Geometry: final body of the model. Coordinates: model frame, mm. Face numbers are marked on the shaded views. Give positions to 0.01 mm unless a question says otherwise; leave off trailing zeros. Write each loop counter-clockwise with the first axis right and the second up, starting at its lowest first coordinate (ties: lowest second). Pieces come first, ordered by that corner, then holes. Notation, with made-up numbers: M -8.75,77.5 L 49.25,77.5 A3 cw 49.25,81.5 Z; hole C 75,-3 d11. An arc over 180 degrees is marked long. Use a Markdown table: item, result. Add a question column.
(1) Pin query (flat end, axial travel): pin 1 Ø6 at (x, y) = (1506.11, -138.7) entering from +Z (3 decimals); pin 2 Ø1 at (x, z) = (1473, 2) entering from +Y; pin 3 Ø1 at (x, z) = (1458.5, 8) entering from +Y; pin 4 Ø3 at (x, y) = (1506.11, -23.75) entering from +Z. Return the tip coordinate at first contact, or that it passes through.
(2) Cut plane B-B (y = -94.5). Output: boundary loops of the cut face in (x, z) (3 decimals), plus the area to 3 significant figures.
(3) Cut plane D-D (y = -14). Output: boundary loops of the cut face in (x, z) (3 decimals), plus the area to 3 significant figures.
(4) Cut plane A-A (z = 5.5). Output: boundary loops of the cut face in (x, y), plus the area to 3 significant figures.
(5) Draft query along Y for the marked faces 1 and 2. Return one class per face: released by +Y, released by -Y, zero draft, split by the parting line, or undercut.
(6) Material intervals for L1, parallel to Y at x = 1467.5, z = 2.25; L2, parallel to X at y = -38, z = 3; L3, parallel to Z at x = 1558, y = -60 (3 decimals), sorted ascending.
(7) Cut plane C-C (x = 1491.5). Output: boundary loops of the cut face in (y, z) (3 decimals).
```python
from build123d import *

# Parameters (mm, degrees)
SKETCH1_W           = 108.712
SKETCH1_H           = 108.712
SKETCH1_R           = 2.54
SKETCH1_R_2         = 3.175
SKETCH1_W_2         = 83.312
SKETCH1_H_2         = 83.312
SKETCH1_R_3         = 0.94996
SKETCH1_R_4         = 0.95
BOSS_EXTRUDE1_DEPTH = 3.175
SKETCH2_R           = 2.54
SKETCH2_R_2         = 0.95
BOSS_EXTRUDE2_DEPTH = 6.35
SKETCH3_R           = 2.54
BOSS_EXTRUDE3_DEPTH = 3.175


with BuildPart() as part:
    # Sketch1 → Boss-Extrude1 (new body)
    # profile 1 of 9: a face of its own
    with BuildSketch(Plane.XY):
        with Locations((1506.110862596, -71.75697427)):
            Rectangle(SKETCH1_W, SKETCH1_H)
        with Locations((1506.110862596, -23.75097427)):
            Circle(SKETCH1_R, mode=Mode.SUBTRACT)
        with Locations((1458.104862596, -23.75097427)):
            Circle(SKETCH1_R_2, mode=Mode.SUBTRACT)
        with Locations((1506.110862596, -119.76297427)):
            Circle(SKETCH1_R, mode=Mode.SUBTRACT)
        with Locations((1554.116862596, -71.75697427)):
            Circle(SKETCH1_R, mode=Mode.SUBTRACT)
        with Locations((1458.104862596, -71.75697427)):
            Circle(SKETCH1_R, mode=Mode.SUBTRACT)
        with Locations((1458.104862596, -119.76297427)):
            Circle(SKETCH1_R, mode=Mode.SUBTRACT)
        with Locations((1554.116862596, -119.76297427)):
            Circle(SKETCH1_R, mode=Mode.SUBTRACT)
        with Locations((1554.116862596, -23.75097427)):
            Circle(SKETCH1_R, mode=Mode.SUBTRACT)
        with Locations((1506.110862596, -71.75697427)):
            Rectangle(SKETCH1_W_2, SKETCH1_H_2, mode=Mode.SUBTRACT)
    # profile 2 of 9: a face of its own
    with BuildSketch(Plane.XY):
        with Locations((1554.116862596, -119.76297427)):
            Circle(SKETCH1_R)
        with Locations((1554.116862596, -119.76297427)):
            Circle(SKETCH1_R_3, mode=Mode.SUBTRACT)
    # profile 3 of 9: a face of its own
    with BuildSketch(Plane.XY):
        with Locations((1554.116862596, -119.76297427)):
            Circle(SKETCH1_R_3)
    # profile 4 of 9: a face of its own
    with BuildSketch(Plane.XY):
        with Locations((1458.104862596, -119.76297427)):
            Circle(SKETCH1_R)
        with Locations((1458.104862596, -119.76297427)):
            Circle(SKETCH1_R_3, mode=Mode.SUBTRACT)
    # profile 5 of 9: a face of its own
    with BuildSketch(Plane.XY):
        with Locations((1458.104862596, -119.76297427)):
            Circle(SKETCH1_R_3)
    # profile 6 of 9: a face of its own
    with BuildSketch(Plane.XY):
        with Locations((1458.104862596, -23.75097427)):
            Circle(SKETCH1_R_2)
        with Locations((1458.104862596, -23.75097427)):
            Circle(SKETCH1_R_4, mode=Mode.SUBTRACT)
    # profile 7 of 9: a face of its own
    with BuildSketch(Plane.XY):
        with Locations((1458.104862596, -23.75097427)):
            Circle(SKETCH1_R_4)
    # profile 8 of 9: a face of its own
    with BuildSketch(Plane.XY):
        with Locations((1554.116862596, -23.75097427)):
            Circle(SKETCH1_R)
        with Locations((1554.116862596, -23.75097427)):
            Circle(SKETCH1_R_3, mode=Mode.SUBTRACT)
    # profile 9 of 9: a face of its own
    with BuildSketch(Plane.XY):
        with Locations((1554.116862596, -23.75097427)):
            Circle(SKETCH1_R_3)
    extrude(amount=BOSS_EXTRUDE1_DEPTH)

    # Sketch2 → Boss-Extrude2 (add)
    # profile 1 of 4: a face of its own
    with BuildSketch(Plane.XY.offset(3.175)):
        with Locations((1554.116862596, -119.76297427)):
            Circle(SKETCH2_R)
        with Locations((1554.116862596, -119.76297427)):
            Circle(SKETCH2_R_2, mode=Mode.SUBTRACT)
    # profile 2 of 4: a face of its own
    with BuildSketch(Plane.XY.offset(3.175)):
        with Locations((1554.116862596, -23.75097427)):
            Circle(SKETCH2_R)
        with Locations((1554.116862596, -23.75097427)):
            Circle(SKETCH2_R_2, mode=Mode.SUBTRACT)
    # profile 3 of 4: a face of its own
    with BuildSketch(Plane.XY.offset(3.175)):
        with Locations((1458.104862596, -23.75097427)):
            Circle(SKETCH2_R)
        with Locations((1458.104862596, -23.75097427)):
            Circle(SKETCH2_R_2, mode=Mode.SUBTRACT)
    # profile 4 of 4: a face of its own
    with BuildSketch(Plane.XY.offset(3.175)):
        with Locations((1458.104862596, -119.76297427)):
            Circle(SKETCH2_R)
        with Locations((1458.104862596, -119.76297427)):
            Circle(SKETCH2_R_2, mode=Mode.SUBTRACT)
    extrude(amount=BOSS_EXTRUDE2_DEPTH)

    # Sketch3 → Boss-Extrude3 (add)
    # profile 1 of 4: a face of its own
    with BuildSketch(Plane.XY.offset(3.175)):
        with BuildLine():
            Line((1513.299858853, -3.795295248), (1515.613291339, -17.40097427))
            Line((1515.613291339, -17.40097427), (1497.000613972, -17.40097427))
            Line((1497.000613972, -17.40097427), (1498.967188582, -3.941668388))
            ThreePointArc((1498.967188582, -3.941668388), (1501.097595235, -0.05597519), (1505.250472182, 1.490264506))
            Line((1505.250472182, 1.490264506), (1506.110862596, 1.490264506))
            Line((1506.110862596, 1.490264506), (1507.039709736, 1.490264506))
            ThreePointArc((1507.039709736, 1.490264506), (1511.136251231, -0.007844339), (1513.299858853, -3.795295248))
        make_face()
        with Locations((1506.110862596, -4.818719074)):
            Circle(SKETCH3_R, mode=Mode.SUBTRACT)
    # profile 2 of 4: a face of its own
    with BuildSketch(Plane.XY.offset(3.175)):
        with BuildLine():
            Line((1432.86362382, -71.75697427), (1432.86362382, -70.82812713))
            ThreePointArc((1432.86362382, -70.82812713), (1434.361732665, -66.731585635), (1438.149183574, -64.567978013))
            Line((1438.149183574, -64.567978013), (1451.754862596, -62.254545527))
            Line((1451.754862596, -62.254545527), (1451.754862596, -80.867222895))
            Line((1451.754862596, -80.867222895), (1438.295556714, -78.900648284))
            ThreePointArc((1438.295556714, -78.900648284), (1434.409863516, -76.770241631), (1432.86362382, -72.617364684))
            Line((1432.86362382, -72.617364684), (1432.86362382, -71.75697427))
        make_face()
        with Locations((1439.1726074, -71.75697427)):
            Circle(SKETCH3_R, mode=Mode.SUBTRACT)
    # profile 3 of 4: a face of its own
    with BuildSketch(Plane.XY.offset(3.175)):
        with BuildLine():
            Line((1574.072541618, -78.945970527), (1560.466862596, -81.259403013))
            Line((1560.466862596, -81.259403013), (1560.466862596, -62.646725646))
            Line((1560.466862596, -62.646725646), (1573.926168478, -64.613300257))
            ThreePointArc((1573.926168478, -64.613300257), (1577.811861676, -66.743706909), (1579.358101372, -70.896583856))
            Line((1579.358101372, -70.896583856), (1579.358101372, -71.75697427))
            Line((1579.358101372, -71.75697427), (1579.358101372, -72.68582141))
            ThreePointArc((1579.358101372, -72.68582141), (1577.859992527, -76.782362905), (1574.072541618, -78.945970527))
        make_face()
        with Locations((1573.049117792, -71.75697427)):
            Circle(SKETCH3_R, mode=Mode.SUBTRACT)
    # profile 4 of 4: a face of its own
    with BuildSketch(Plane.XY.offset(3.175)):
        with BuildLine():
            Line((1498.921866339, -139.718653293), (1496.608433853, -126.11297427))
            Line((1496.608433853, -126.11297427), (1515.22111122, -126.11297427))
            Line((1515.22111122, -126.11297427), (1513.254536609, -139.572280152))
            ThreePointArc((1513.254536609, -139.572280152), (1511.124129957, -143.45797335), (1506.97125301, -145.004213046))
            Line((1506.97125301, -145.004213046), (1506.110862596, -145.004213046))
            Line((1506.110862596, -145.004213046), (1505.182015456, -145.004213046))
            ThreePointArc((1505.182015456, -145.004213046), (1501.085473961, -143.506104201), (1498.921866339, -139.718653293))
        make_face()
        with Locations((1506.110862596, -138.695229466)):
            Circle(SKETCH3_R, mode=Mode.SUBTRACT)
    extrude(amount=-BOSS_EXTRUDE3_DEPTH)


solid = part.part
```
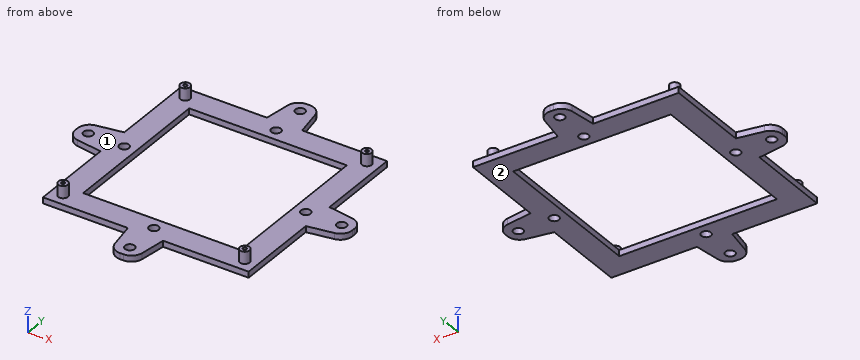
Answer list:
| question | item | result |
|---|---|---|
| 1 | pin 1 | z = 3.175 |
| 1 | pin 2 | y = -17.4 |
| 1 | pin 3 | y = -21.21 |
| 1 | pin 4 | through |
| 2 | outline | M 1451.755,0 L 1464.455,0 L 1464.455,3.175 L 1451.755,3.175 Z; M 1547.767,0 L 1560.467,0 L 1560.467,3.175 L 1547.767,3.175 Z |
| 2 | area | 80.6 mm² |
| 3 | outline | M 1497.498,0 L 1515.035,0 L 1515.035,3.175 L 1497.498,3.175 Z |
| 3 | area | 55.7 mm² |
| 4 | outline | C 1458.1,-119.76 d5.08; C 1458.1,-23.75 d5.08; C 1554.12,-119.76 d5.08; C 1554.12,-23.75 d5.08; hole C 1458.1,-119.76 d1.9; hole C 1458.1,-23.75 d1.9; hole C 1554.12,-119.76 d1.9; hole C 1554.12,-23.75 d1.9 |
| 4 | area | 69.7 mm² |
| 5 | face 1 | undercut |
| 5 | face 2 | zero draft |
| 6 | L1 | -126.11 to -113.41, -30.1 to -17.4 |
| 6 | L2 | 1451.75 to 1464.45, 1547.77 to 1560.47 |
| 6 | L3 | 0 to 3.175 |
| 7 | outline | M -126.113,0 L -113.413,0 L -113.413,3.175 L -126.113,3.175 Z; M -30.101,0 L -17.401,0 L -17.401,3.175 L -30.101,3.175 Z |
